Autodesk Inventor part; units mm, degrees
ref_plane "YZ Plane" through (0, 0, 0) normal (1, 0, 0) x (0, 1, 0)
ref_plane "XZ Plane" through (0, 0, 0) normal (0, 1, 0) x (-1, 0, 0)
ref_plane "XY Plane" through (0, 0, 0) normal (0, 0, 1) x (1, 0, 0)
sketch "Sketch1" plane through (0, 0, 0) normal (0, 0, 1) x (1, 0, 0)
  line L0 (-50, 50) -> (50, 50)
  line L1 (50, 50) -> (50, -50)
  line L2 (50, -50) -> (-50, -50)
  line L3 (-50, -50) -> (-50, 50)
  line L4 (-92.7646, -8.503) -> (-89.7646, -8.503)
  line L5 (-89.7646, -8.503) -> (-89.7646, -11.753)
  line L6 (-89.7646, -11.753) -> (-92.7646, -11.753)
  line L7 (-92.7646, -11.753) -> (-92.7646, -8.503)
  line L8 (-92.7646, -21.6527) -> (-89.7646, -21.6527)
  line L9 (-89.7646, -21.6527) -> (-89.7646, -21.7527)
  line L10 (-89.7646, -21.7527) -> (-92.7646, -21.7527)
  line L11 (-92.7646, -21.7527) -> (-92.7646, -21.6527)
  line L12 (-50, 50) -> (-46.75, 50)
  line L13 (-46.75, 50) -> (-46.75, 36)
  line L14 (-46.75, 36) -> (-50, 36)
  line L15 (-50, 36) -> (-50, 50)
  line L16 (0, 50) -> (0, -50) construction
  line L17 (-50, 0) -> (50, 0) construction
  line L18 (50, 50) -> (46.75, 50)
  line L19 (46.75, 50) -> (46.75, 36)
  line L20 (46.75, 36) -> (50, 36)
  line L21 (50, 36) -> (50, 50)
  line L22 (-50, -50) -> (-46.75, -50)
  line L23 (-46.75, -50) -> (-46.75, -36)
  line L24 (-46.75, -36) -> (-50, -36)
  line L25 (-50, -36) -> (-50, -50)
  line L26 (46.75, -50) -> (46.75, -36)
  line L27 (46.75, -36) -> (50, -36)
  line L28 (50, -36) -> (50, -50)
  line L29 (50, -50) -> (46.75, -50)
  line L30 (-40, 40) -> (-10, 40)
  line L31 (-10, 40) -> (-10, 0)
  line L32 (-10, 0) -> (-40, 0)
  line L33 (-40, 0) -> (-40, 40)
  line L34 (40, 40) -> (10, 40)
  line L35 (10, 40) -> (10, 0)
  line L36 (10, 0) -> (40, 0)
  line L37 (40, 0) -> (40, 40)
  line L38 (-10, 50) -> (-6.75, 50)
  line L39 (-6.75, 50) -> (-6.75, 42)
  line L40 (-6.75, 42) -> (-10, 42)
  line L41 (-10, 42) -> (-10, 50)
  line L42 (10, 50) -> (6.75, 50)
  line L43 (6.75, 50) -> (6.75, 42)
  line L44 (6.75, 42) -> (10, 42)
  line L45 (10, 42) -> (10, 50)
  line L46 (-25, 0) -> (-25, 40) construction
  line L47 (-40, 50) -> (-43.25, 50)
  line L48 (-43.25, 50) -> (-43.25, 42)
  line L49 (-43.25, 42) -> (-40, 42)
  line L50 (-40, 42) -> (-40, 50)
  line L51 (43.25, 42) -> (40, 42)
  line L52 (43.25, 50) -> (43.25, 42)
  line L53 (40, 50) -> (43.25, 50)
  line L54 (40, 42) -> (40, 50)
  line L55 (-20, -15) -> (20, -15)
  line L56 (20, -15) -> (20, -30)
  line L57 (20, -30) -> (-20, -30)
  line L58 (-20, -30) -> (-20, -15)
  line L59 (-25, -10) -> (25, -10)
  line L60 (25, -10) -> (25, -35)
  line L61 (25, -35) -> (-25, -35)
  line L62 (-25, -35) -> (-25, -10)
  line L63 (0, -15) -> (0, -30) construction
  line L64 (-5, -10) -> (5, -10)
  line L65 (5, -10) -> (5, 62)
  line L66 (5, 62) -> (-5, 62)
  line L67 (-5, 62) -> (-5, -10)
  line L68 (0, 62) -> (0, -10) construction
  line L69 (-17.5, 62) -> (17.5, 62)
  line L70 (17.5, 62) -> (17.5, 76)
  line L71 (17.5, 76) -> (-17.5, 76)
  line L72 (-17.5, 76) -> (-17.5, 62)
  line L73 (0, 76) -> (0, 62) construction
  line L74 (-20, -22.5) -> (20, -22.5) construction
  line L75 (-12.5, 72.5) -> (-9.25, 72.5)
  line L76 (-9.25, 72.5) -> (-9.25, 65.5)
  line L77 (-9.25, 65.5) -> (-12.5, 65.5)
  line L78 (-12.5, 65.5) -> (-12.5, 72.5)
  line L79 (-12.5, 69) -> (-9.25, 69) construction
  line L80 (12.5, 72.5) -> (9.25, 72.5)
  line L81 (9.25, 72.5) -> (9.25, 65.5)
  line L82 (9.25, 65.5) -> (12.5, 65.5)
  line L83 (12.5, 65.5) -> (12.5, 72.5)
  line L84 (12.5, 69) -> (9.25, 69) construction
  point P0 (0, 0)
  dimension "d0" = 100
  dimension "d2" = 100
  dimension "d3" = 3
  dimension "mat" = 3.25
  dimension "d5" = 3
  dimension "kerf" = 0.1
  dimension "d7" = 3.25
  dimension "d8" = 14
  dimension "d9" = 30
  dimension "d10" = 40
  dimension "d11" = 10
  dimension "d12" = 10
  dimension "d15" = 3.25
  dimension "d16" = 8
  dimension "d17" = 0
  dimension "d22" = 40
  dimension "d23" = 15
  dimension "d24" = 5
  dimension "d25" = 5
  dimension "d26" = 5
  dimension "d27" = 5
  dimension "d28" = 15
  dimension "d29" = 72
  dimension "d30" = 14
  dimension "d31" = 10
  dimension "d32" = 35
  dimension "d35" = 27.5
  dimension "d36" = 3.25
  dimension "d37" = 7
  dimension "d38" = 7
  dimension "d39" = 5
extrude "Extrusion4" add sketch "Sketch1" along normal blind 3.25 contours L67 L66 L65 L0 | L0 L65 L59 L67 | L69 L72 L71 L70 L66 | L59 L60 L61 L62 | L75 L76 L77 L78 | L83 L82 L81 L80
extrude "Extrusion5" cut sketch "Sketch1" along normal blind 3.25 contours L75 L76 L77 L78 | L83 L82 L81 L80
equation "\"d7\" = mat"
equation "\"d15\" = mat"
equation "\"d36\" = mat"
equation "\"d33\" = mat"
equation "\"d40\" = mat"
properties part number "body-back"
Input: part model. Units: mm. Frame: model coordinates. A direction names the side the tool comes from. Round coordinates to 2 decimals unless told otherwise and drop trailing zeros. Loops run counter-clockwise (first coordinate to the right, second up) from the corner with the lowest first, then second, coordinate; pieces in that order, holes last. Notation, with made-up numbers: (-35.75, 88) -> (22.25, 88) arc R14 cw to (22.25, 114) -> close; hole circle Ø7 at (-24, 14). An arc over 180 degrees is marked (long way). One line per item, written item: value.
(1) Mould query, pull axis X, two halves, no side actions, for faces 4 (the face through (-12.5, 69, 2)), 5 (the face through (0, 17, 0)), 6 (the face through (5, 25, 2)), 7 (the face through (-25, -23, 2)). Classes: pulls with the +X half, pulls with the -X half, needs draft (parallel to the pull), parting line crosses it, or undercut.
Geometry check:
face 4: undercut
face 5: needs draft
face 6: pulls with the +X half
face 7: pulls with the -X half
(2) Set-up query: faces 1 (the face through (-15, -10, 2)), 2 (the face through (17.5, 69, 2)), 3 (the face through (11, 62, 2)). Return all of +Z, -Z, +X, -X, +Y, -Y with unobstructed straight access to the full face (end or side cutting, diameter ignored); none if empty.
Geometry check:
face 1: +Z, -Z, -X
face 2: +Z, -Z, +X, +Y
face 3: +Z, -Z, +X
(3) Section B-B (z = 1.4). Return the cut outline in (x, y), plus the area to 3 significant figures.
Geometry check:
outline: (-25, -35) -> (25, -35) -> (25, -10) -> (5, -10) -> (5, 62) -> (17.5, 62) -> (17.5, 76) -> (-17.5, 76) -> (-17.5, 62) -> (-5, 62) -> (-5, -10) -> (-25, -10) -> close; hole (-20, -30) -> (20, -30) -> (20, -15) -> (-20, -15) -> close; hole (-12.5, 65.5) -> (-9.25, 65.5) -> (-9.25, 72.5) -> (-12.5, 72.5) -> close; hole (9.25, 65.5) -> (12.5, 65.5) -> (12.5, 72.5) -> (9.25, 72.5) -> close
area: 1,810 mm2
(4) Material intervals for line 1 (Y direction, x = 8.5, z = 2.15); line 2 (X direction, y = 69.5, z = 0.85); line 3 (Y direction, x = -4.5, z = 0.7), sorted ascending. Write a range as [from, to].
Geometry check:
line 1: [-35, -30], [-15, -10], [62, 76]
line 2: [-17.5, -12.5], [-9.25, 9.25], [12.5, 17.5]
line 3: [-35, -30], [-15, 76]
(5) Section D-D (y = -5). Return the cut outline in (x, z).
Geometry check:
outline: (-5, 0) -> (5, 0) -> (5, 3.25) -> (-5, 3.25) -> close
(6) Pin query (flat end, axial travel): pin 1 (1.6 mm diameter, centred on y = 69, z = 1.5, fed in from +X); pin 2 (1.6 mm diameter, centred on y = 15, z = 2.5, fed in from +X); pin 3 (1.6 mm diameter, centred on y = 68, z = 2, fed in from -X). Return the tip coordinate at first contact, or that it passes through.
Geometry check:
pin 1: x = 17.5
pin 2: x = 5
pin 3: x = -17.5
(7) Section A-A (x = 4). Return the cut outline in (y, z).
Geometry check:
outline: (-35, 0) -> (-30, 0) -> (-30, 3.25) -> (-35, 3.25) -> close; (-15, 0) -> (76, 0) -> (76, 3.25) -> (-15, 3.25) -> close
(8) Section C-C (x = 19). Return the cut outline in (y, z).
Geometry check:
outline: (-35, 0) -> (-30, 0) -> (-30, 3.25) -> (-35, 3.25) -> close; (-15, 0) -> (-10, 0) -> (-10, 3.25) -> (-15, 3.25) -> close
